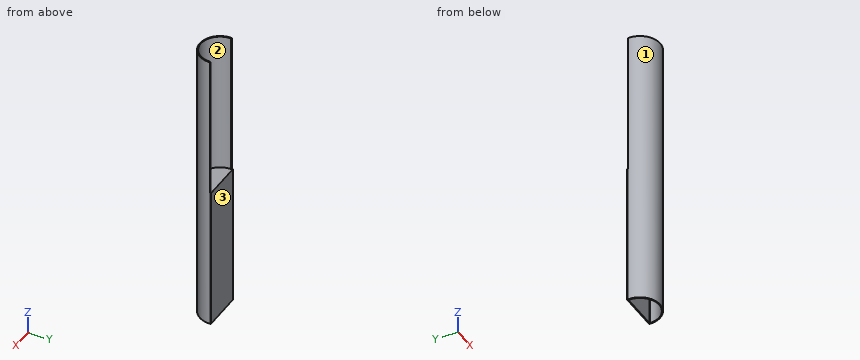
```python
from build123d import *

# Parameters (mm, degrees)
BOSS_EXTRUDE1_DEPTH = 600
SKETCH2_W           = 83.904707854
SKETCH2_H           = 300
BOSS_EXTRUDE2_DEPTH = 2
BOSS_EXTRUDE3_START = -298
BOSS_EXTRUDE3_DEPTH = 2


with BuildPart() as part:
    # Sketch1 → Boss-Extrude1 (new body)
    with BuildSketch(Plane.XY):
        with BuildLine():
            Line((41.952353927, 2), (40, 2))
            Line((40, 2), (40, 0))
            ThreePointArc((40, 0), (0, -40), (-40, 0))
            Line((-40, 0), (-40, 2))
            Line((-40, 2), (-41.952353927, 2))
            ThreePointArc((-41.952353927, 2), (0, -42), (41.952353927, 2))
        make_face()
    extrude(amount=BOSS_EXTRUDE1_DEPTH)

    # Sketch2 → Boss-Extrude2 (add)
    with BuildSketch(Plane(origin=(0, 2, 0), x_dir=(1, 0, 0), z_dir=(0, 1, 0))):
        with Locations((0, -150)):
            Rectangle(SKETCH2_W, SKETCH2_H)
    extrude(amount=BOSS_EXTRUDE2_DEPTH)

    # Sketch3 → Boss-Extrude3 (add)
    with BuildSketch(Plane(origin=(0, 0, 0), x_dir=(-1, 0, 0), z_dir=(0, 0, -1)).offset(BOSS_EXTRUDE3_START)):
        with BuildLine():
            Line((41.952353927, 2), (-41.952353927, 2))
            ThreePointArc((-41.952353927, 2), (0, -42), (41.952353927, 2))
        make_face()
    extrude(amount=-BOSS_EXTRUDE3_DEPTH)


solid = part.part
```
Geometry: final body of the model. Coordinates: model frame, mm. Face numbers are marked on the shaded views. Coordinates: 2 decimals unless noted, no trailing zeros. Order: outer loops, then holes, each group sorted by start corner. A loop starts at its lowest first (then second) coordinate and runs counter-clockwise, first axis right, second up. Notation, with made-up numbers: M 56,-2.75 L 90,-2.75 A29 ccw 90,22.25 Z; hole C 21.25,49 d3. An arc over 180 degrees is marked long. Answer in a Markdown table with one row per item. Add a question column.
Q1. Section query A-A on x = 0. Return the cut outline in (y, z).
Q2. Section query C-C on y = -32.5. Return the cut outline in (x, z), and give its area (3 significant figures).
Q3. Contact query for flat-ended pins moving along their axis: P1, Ø1, axis at x = 4, y = -20.5, coming from the +Z side; P2, Ø1.6, axis at y = 1.5, z = 222.5, coming from the -X side; P3, Ø0.6, axis at y = 3, z = 155, coming from the +X side; P4, Ø1.5, axis at x = -30.5, y = -27.5, coming from the -Z side. Output: stop coordinate, or through.
Q4. Line query: L1, parallel to X at y = 0, z = 432; L2, parallel to Y at x = 2.5, z = 251; L3, parallel to Z at x = -24, y = -3.5. Output: solid intervals per line, ascending.
Q5. Mould query, pull axis X, two halves, no side actions, for the marked faces 1, 2 and 3. Classes: released by +X, released by -X, zero draft, split by the parting line, or undercut.
Q6. Section query B-B on z = 237. Return the cut outline in (x, y), and give its area (3 significant figures).
Completed:
| question | item | result |
|---|---|---|
| 1 | outline | M -42,0 L -40,0 L -40,298 L 2,298 L 2,0 L 4,0 L 4,300 L -40,300 L -40,600 L -42,600 Z |
| 2 | outline | M -26.6,0 L -23.32,0 L -23.32,298 L 23.32,298 L 23.32,0 L 26.6,0 L 26.6,600 L 23.32,600 L 23.32,300 L -23.32,300 L -23.32,600 L -26.6,600 Z |
| 2 | area | 4,040 mm2 |
| 3 | P1 | stops at z = 300 |
| 3 | P2 | stops at x = -41.99 |
| 3 | P3 | stops at x = 41.95 |
| 3 | P4 | stops at z = 0 |
| 4 | L1 | x = -42 to -40, 40 to 42 |
| 4 | L2 | y = -41.93 to -39.92, 2 to 4 |
| 4 | L3 | z = 298 to 300 |
| 5 | face 1 | split by the parting line |
| 5 | face 2 | undercut |
| 5 | face 3 | zero draft |
| 6 | outline | M -41.95,2 A42 ccw long 41.95,2 L 41.95,4 L -41.95,4 Z; hole M -40,0 A40 ccw 40,0 L 40,2 L -40,2 Z |
| 6 | area | 433 mm2 |
